Part model, mm, in its own coordinate system. Face numbers are marked on the shaded views. A direction names the side the tool comes from. Give positions to 0.01 mm unless a question says otherwise; leave off trailing zeros. Order: outer loops, then holes, each group sorted by start corner. A loop starts at its lowest first (then second) coordinate and runs counter-clockwise, first axis right, second up. Notation, with made-up numbers: (81.5, -13) - (86.5, -13) arc R22 ccw to (86.5, 18) - close; hole circle Ø2 at (8.5, -37). An arc over 180 degrees is marked (long way). Use one line per item in the form item = value. Start each with the question number.
1. Band-saw the part on D-D, the plane z = 44. List the corners of the cut face in (x, y).
2. Pin check, flat tips, straight feed: P1, Ø10, axis at x = 137.5, z = 49, coming from the +Y side; P2, Ø24, axis at x = 11.5, y = 60, coming from the -Z side; P3, Ø8, axis at x = 27.5, y = -23.5, coming from the +Z side; P4, Ø4, axis at x = 18, z = 67, coming from the +Y side. Stop position of each tip, or through.
3. Pull direction Y, two halves, no side cores. Call the marked faces 1, 2 and 3: +Y half, -Y half, draft (parallel to the pull), parting line (faces both ways), or undercut.
4. Drill centre lines: line 1 (X direction, y = -1, z = 67); line 2 (Y direction, x = 217, z = -3); line 3 (X direction, y = 70.5, z = 70.5). Where is each one in solid material? Low to high.
5. Band-saw the part on A-A, the plane y = 66. List the corners of the cut face in (x, z).
6. Tool access for the marked faces 4, 5 and 6: list every direction of +Z, -Z, +X, -X, +Y, -Y with a clear straight run to the whole face (end or side of a thin tool).
7. Band-saw the part on B-B, the plane z = 13.5. List the corners of the cut face in (x, y).
8. Band-saw the part on C-C, the plane x = 61. List the corners of the cut face in (y, z), plus the area to 3 significant figures.
from build123d import *

# Parameters (mm, degrees)
SKETCH1_W           = 260
SKETCH1_H           = 80
BOSS_EXTRUDE1_DEPTH = 80
SHELL1_T            = 2
SKETCH3_W           = 30
SKETCH3_H           = 170
BOSS_EXTRUDE2_DEPTH = 5
SKETCH4_R           = 5
CUT_EXTRUDE3_DEPTH  = 7
SKETCH6_R           = 13
CUT_EXTRUDE4_DEPTH  = 2
SKETCH7_R           = 2.5
CUT_EXTRUDE5_DEPTH  = 82


with BuildPart() as part:
    # Sketch1 → Boss-Extrude1 (new body)
    with BuildSketch(Plane.XY):
        with Locations((130, 40)):
            Rectangle(SKETCH1_W, SKETCH1_H)
    extrude(amount=BOSS_EXTRUDE1_DEPTH)

    # Shell1
    shell1_openings = [part.faces().sort_by_distance(p)[0] for p in [
        (130, 40, 80),
    ]]
    offset(amount=SHELL1_T, openings=shell1_openings, kind=Kind.INTERSECTION)

    # Sketch3 → Boss-Extrude2 (add)
    with BuildSketch(Plane(origin=(0, 0, -2), x_dir=(-1, 0, 0), z_dir=(0, 0, -1))):
        with Locations((-217, 40)):
            Rectangle(SKETCH3_W, SKETCH3_H)
        with Locations((-43, 40)):
            Rectangle(SKETCH3_W, SKETCH3_H)
    extrude(amount=BOSS_EXTRUDE2_DEPTH)

    # Sketch4 → Cut-Extrude3 (cut)
    with BuildSketch(Plane(origin=(0, 0, -7), x_dir=(-1, 0, 0), z_dir=(0, 0, -1))):
        with Locations((-217, 66)):
            Circle(SKETCH4_R)
        with Locations((-217, 14)):
            Circle(SKETCH4_R)
    cut_extrude3 = extrude(amount=-CUT_EXTRUDE3_DEPTH, mode=Mode.SUBTRACT)

    # Mirror1: Cut-Extrude3 across plane
    add(cut_extrude3.mirror(Plane(origin=(130, 0, 0), x_dir=(0, 0, 1), z_dir=(1, 0, 0))), mode=Mode.SUBTRACT)

    # Sketch6 → Cut-Extrude4 (cut)
    with BuildSketch(Plane(origin=(0, 82, 0), x_dir=(1, 0, 0), z_dir=(0, 1, 0))):
        with Locations(Location((222, -40, 0), (0, 0, 270))):
            Circle(SKETCH6_R)
    extrude(amount=-CUT_EXTRUDE4_DEPTH, mode=Mode.SUBTRACT)

    # Sketch7 → Cut-Extrude5 (cut)
    with BuildSketch(Plane(origin=(0, 82, 0), x_dir=(1, 0, 0), z_dir=(0, 1, 0))):
        with Locations(Location((18, -67, 0), (0, 0, 270))):
            Circle(SKETCH7_R)
        with Locations(Location((242, -67, 0), (0, 0, 270))):
            Circle(SKETCH7_R)
    cut_extrude5 = extrude(amount=-CUT_EXTRUDE5_DEPTH, mode=Mode.SUBTRACT)

    # Mirror2: Cut-Extrude5 across plane
    add(cut_extrude5.mirror(Plane(origin=(0, 40, 0), x_dir=(0, 0, 1), z_dir=(0, -1, 0))), mode=Mode.SUBTRACT)


solid = part.part
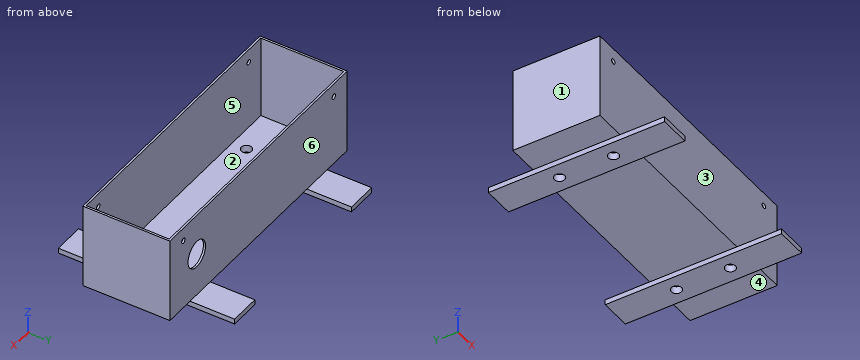
From the geometry:
q1.outline = (-2, -2) - (262, -2) - (262, 82) - (234.37, 82) - (234.37, 80) - (260, 80) - (260, 0) - (0, 0) - (0, 80) - (209.63, 80) - (209.63, 82) - (-2, 82) - close
q2.P1 = 82
q2.P2 = -2
q2.P3 = -2
q2.P4 = through
q3.face_1 = draft
q3.face_2 = undercut
q3.face_3 = -Y half
q4.line_1 = -2 to 15.5, 20.5 to 239.5, 244.5 to 262
q4.line_2 = -45 to 9, 19 to 61, 71 to 125
q4.line_3 = -2 to 0, 260 to 262
q5.outline = (-2, -2) - (28, -2) - (28, -7) - (38, -7) - (38, 0) - (0, 0) - (0, 80) - (-2, 80) - close; (48, -7) - (58, -7) - (58, -2) - (202, -2) - (202, -7) - (212, -7) - (212, 0) - (48, 0) - close; (222, -7) - (232, -7) - (232, -2) - (262, -2) - (262, 80) - (260, 80) - (260, 0) - (222, 0) - close
q6.face_4 = -Z, +X, +Y, -Y
q6.face_5 = +Z
q6.face_6 = +Z, +X, -X, +Y
q7.outline = (-2, -2) - (262, -2) - (262, 82) - (-2, 82) - close; hole (0, 0) - (260, 0) - (260, 80) - (0, 80) - close
q8.outline = (-2, -2) - (82, -2) - (82, 80) - (80, 80) - (80, 0) - (0, 0) - (0, 80) - (-2, 80) - close
q8.area = 488 mm²
